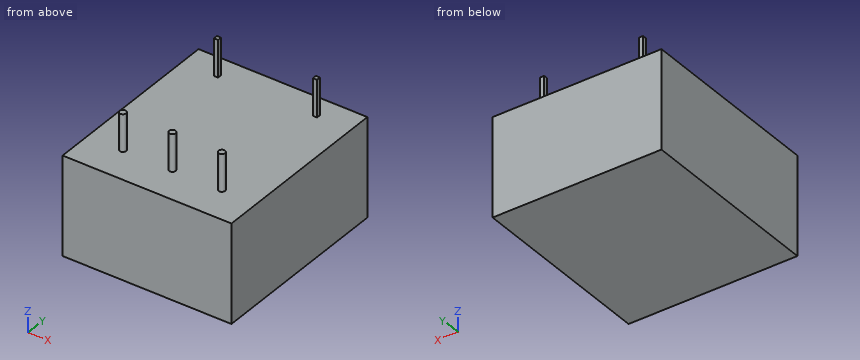
from build123d import *

# Parameters (mm, degrees)
SKETCH_W         = 26
SKETCH_H         = 29.2
EXTRUDE_DEPTH    = 15.2
SKETCH001_R      = 0.5
SKETCH001_W      = 0.635
SKETCH001_H      = 0.635
EXTRUDE001_DEPTH = 5.7


with BuildPart() as extrude_body:
    # Sketch → Extrude (new body)
    with BuildSketch(Plane.XY):
        with Locations((-7.62, -11.16)):
            Rectangle(SKETCH_W, SKETCH_H)
    extrude(amount=-EXTRUDE_DEPTH)


with BuildPart() as fusion:
    # Sketch001 → Extrude001 (new body)
    with BuildSketch(Plane.XY):
        with Locations((-15.24, -20.32)):
            Circle(SKETCH001_R)
        with Locations((-7.62, -20.32)):
            Circle(SKETCH001_R)
        with Locations((0, -20.32)):
            Circle(SKETCH001_R)
        Rectangle(SKETCH001_W, SKETCH001_H)
        with Locations((-15.24, 0)):
            Rectangle(SKETCH001_W, SKETCH001_H)
    extrude(amount=EXTRUDE001_DEPTH)

    # Fusion: union Extrude body
    add(extrude_body.part)


solid = fusion.part
Verification items for the finished model (mm, model axes). Round coordinates to 2 decimals unless told otherwise and drop trailing zeros. Loops run counter-clockwise (first coordinate to the right, second up) from the corner with the lowest first, then second, coordinate; pieces in that order, holes last. Notation, with made-up numbers: (3, 75.5) - (32, 75.5) arc R23 cw to (32, 96.5) - close; hole circle Ø2 at (14.25, 2). An arc over 180 degrees is marked (long way). Use a Markdown table: item, result. Add a question column.
1. Gauge pin test, flat ends, axial feed: pin 1 (13 mm diameter, centred on x = -7, y = -10, fed in from +Z); pin 2 (0.7 mm diameter, centred on x = 0, z = 3.5, fed in from +Y); pin 3 (0.7 mm diameter, centred on y = 0, z = 1.5, fed in from +X). Record the tip position at first contact, or that the pin passes through.
2. Section check B-B, the plane x = -7.62. Record the boundary of the cut face in (y, z).
3. Section check A-A, the plane y = -20.32. Record the boundary of the cut face in (x, z).
4. Section check C-C, the plane x = -1.25. Record the boundary of the cut face in (y, z).
5. Thickness scan on probe 1 along Z at (x, y) = (-9.5, 2.25). Record the ranges inside material, lowest first. Write a range as [from, to].
Checks:
| question | item | result |
|---|---|---|
| 1 | pin 1 | stops at z = 0 |
| 1 | pin 2 | stops at y = 0.32 |
| 1 | pin 3 | stops at x = 0.32 |
| 2 | outline | (-25.76, -15.2) - (3.44, -15.2) - (3.44, 0) - (-19.82, 0) - (-19.82, 5.7) - (-20.82, 5.7) - (-20.82, 0) - (-25.76, 0) - close |
| 3 | outline | (-20.62, -15.2) - (5.38, -15.2) - (5.38, 0) - (0.5, 0) - (0.5, 5.7) - (-0.5, 5.7) - (-0.5, 0) - (-7.12, 0) - (-7.12, 5.7) - (-8.12, 5.7) - (-8.12, 0) - (-14.74, 0) - (-14.74, 5.7) - (-15.74, 5.7) - (-15.74, 0) - (-20.62, 0) - close |
| 4 | outline | (-25.76, -15.2) - (3.44, -15.2) - (3.44, 0) - (-25.76, 0) - close |
| 5 | probe 1 | z = [-15.2, 0] |
